Input: part model. Units: mm. Frame: model coordinates. A direction names the side the tool comes from. Give positions to 0.01 mm unless a question says otherwise; leave off trailing zeros. Write each loop counter-clockwise with the first axis right and the second up, starting at its lowest first coordinate (ties: lowest second). Pieces come first, ordered by that corner, then holes. Notation, with made-up numbers: (18.25, 69) -> (47.25, 69) arc R17 ccw to (47.25, 101) -> close; hole circle Ø8 at (75.5, 45.25). An arc over 180 degrees is marked (long way). Return JSON: item names as keys, results as strings. Group by question number.
Item 1: Mould query, pull axis X, two halves, no side actions, for faces 6 (the face through (-29.167, -16.817, 2.465)), 7 (the face through (0, -12, 0)), 8 (the face through (27.2, -15.64, 2.46)). Classes: released by +X, released by -X, zero draft, split by the parting line, or undercut.
Item 2: Pin query (flat end, axial travel): P1, Ø1.5, axis at x = -19, z = 1, coming from the +Y side. Return the tip coordinate at first contact, or that it passes through.
Item 3: Section A-A, the plane x = 0. Return loops of the section in (y, z).
Item 4: Section B-B, the plane y = 10. Return loops of the section in (x, z), then the cut area to 3 significant figures.
Item 5: Set-up query: faces 1 (the face through (0, -12, 5)), 2 (the face through (-35.053, -8.048, 2.465)), 3 (the face through (-13.57, -18.42, 2.46)), 4 (the face through (-27.15, -15.73, 2.46)), 5 (the face through (22.74, -2.54, 2.46)). Return all of +Z, -Z, +X, -X, +Y, -Y with unobstructed straight access to the full face (end or side cutting, diameter ignored); none if empty.
Item 6: Section C-C, the plane z = 2.85. Count the separate pieces of the cut face and the enclosed holes in it, then the cut area to 3 significant figures.
Item 7: Line query: line 1 (X direction, y = -9.5, z = 0.75); line 2 (X direction, y = -7.5, z = 0.3); line 3 (Y direction, x = 0, z = 2.3). Output: solid intervals per line, ascending. Write a range as [from, to].
from build123d import *

# Parameters (mm, degrees)
F0_R     = 11.8128779822
F1_DEPTH = 5


with BuildPart() as f1:
    # F0 (on Top) → F1 (new body)
    with BuildSketch(Plane.XY):
        with BuildLine():
            ThreePointArc((-10.9877368692, -13.3584800376), (-14.4276328661, -8.4296575195), (-15.7757547816, -2.5722909453))
            ThreePointArc((-15.7757547816, -2.5722909453), (-16.4566838692, -2.7870228586), (-17.1690704864, -2.8347672253))
            Line((-17.1690704864, -2.8347672253), (-28.1587377075, -2.2588231712))
            ThreePointArc((-28.1587377075, -2.2588231712), (-35.0758085793, -8.184518487), (-30.2818924612, -15.9290715842))
            ThreePointArc((-30.2818924612, -15.9290715842), (-29.1564572976, -16.8348568451), (-28.9347418331, -18.2624049175))
            ThreePointArc((-28.9347418331, -18.2624049175), (-24.6247201691, -26.286334608), (-16.0343820545, -23.2588231712))
            Line((-16.0343820545, -23.2588231712), (-11.038330626, -13.4535201515))
            ThreePointArc((-11.038330626, -13.4535201515), (-11.0134601469, -13.4057731047), (-10.9877368692, -13.3584800376))
        make_face()
        Polygon((-29.0074426032, -12.5088231712), (-25.3354948912, -6.1488231712), (-17.9915994671, -6.1488231712), (-14.319651755, -12.5088231712), (-17.9915994671, -18.8688231712), (-25.3354948912, -18.8688231712), align=None, mode=Mode.SUBTRACT)
        with BuildLine():
            ThreePointArc((15.7758429715, -2.5697420135), (15.7828894553, -2.2975080655), (15.7852385163, -2.0251930691))
            ThreePointArc((15.7852385163, -2.0251930691), (13.4879848824, 6.1752958693), (7.264870736, 11.9889215374))
            ThreePointArc((7.264870736, 11.9889215374), (-8.4330311307, 11.3186347537), (-15.7757547816, -2.5722909453))
            ThreePointArc((-15.7757547816, -2.5722909453), (-14.4276328661, -8.4296575195), (-10.9877368692, -13.3584800376))
            ThreePointArc((-10.9877368692, -13.3584800376), (0.0010524985, -17.8104315503), (10.9892480908, -13.3570146974))
            ThreePointArc((10.9892480908, -13.3570146974), (14.4285771261, -8.4275299185), (15.7758429715, -2.5697420135))
        make_face()
        Circle(F0_R, mode=Mode.SUBTRACT)
        with BuildLine():
            ThreePointArc((17.1702555345, -2.8327146617), (16.4572773621, -2.784858795), (15.7758429715, -2.5697420135))
            ThreePointArc((15.7758429715, -2.5697420135), (14.4285771261, -8.4275299185), (10.9892480908, -13.3570146974))
            ThreePointArc((10.9892480908, -13.3570146974), (11.0148030033, -13.4040170233), (11.0395156741, -13.451467588))
            Line((11.0395156741, -13.451467588), (16.0355671026, -23.2567706076))
            ThreePointArc((16.0355671026, -23.2567706076), (24.6259052172, -26.2842820445), (28.9359268812, -18.260352354))
            ThreePointArc((28.9359268812, -18.260352354), (29.1576423457, -16.8328042815), (30.2830775093, -15.9270190207))
            ThreePointArc((30.2830775093, -15.9270190207), (35.0769936274, -8.1824659235), (28.1599227556, -2.2567706076))
            Line((28.1599227556, -2.2567706076), (17.1702555345, -2.8327146617))
        make_face()
        Polygon((25.3366799393, -18.8667706076), (17.9927845152, -18.8667706076), (14.3208368031, -12.5067706076), (17.9927845152, -6.1467706076), (25.3366799393, -6.1467706076), (29.0086276513, -12.5067706076), align=None, mode=Mode.SUBTRACT)
    extrude(amount=F1_DEPTH)


solid = f1.part
Answer below:
{
 "1": {"face 6": "released by -X", "face 7": "zero draft", "face 8": "undercut"},
 "2": {"P1": "stops at y = -2.7"},
 "3": {"outline": "(-17.81, 0) -> (-11.81, 0) -> (-11.81, 5) -> (-17.81, 5) -> close; (11.81, 0) -> (13.76, 0) -> (13.76, 5) -> (11.81, 5) -> close"},
 "4": {"outline": "(-10.23, 0) -> (-6.29, 0) -> (-6.29, 5) -> (-10.23, 5) -> close; (6.29, 0) -> (10.23, 0) -> (10.23, 5) -> (6.29, 5) -> close", "area": "39.4 mm2"},
 "5": {"face 1": "+Z, +X, -X, +Y, -Y", "face 2": "+Z, -Z, -X", "face 3": "+Z, -Z, -Y", "face 4": "+Z, -Z", "face 5": "+Z, -Z, +Y"},
 "6": {"separate pieces": "1", "enclosed holes": "3", "area": "880 mm2"},
 "7": {"line 1": "x = [-35.15, -27.27], [-16.06, -7.02], [7.02, 16.06], [27.27, 35.16]", "line 2": "x = [-34.93, -26.12], [-17.21, -9.13], [9.13, 17.21], [26.12, 34.94]", "line 3": "y = [-17.81, -11.81], [11.81, 13.76]"}
}
